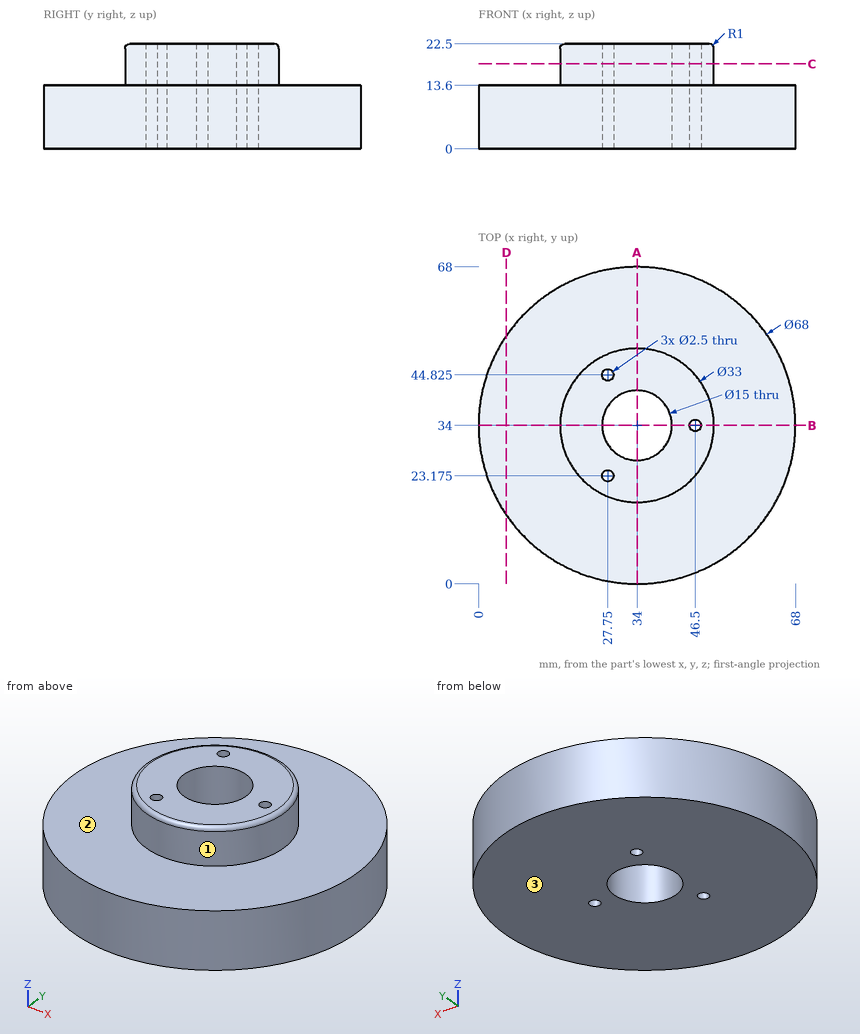
Can you work these out from the drawing? Everything is in mm from the part's minimum corner. Give positions to 0.01 mm unless a question says otherwise; leave off trailing zeros. Order: outer loops, then holes, each group sorted by start corner. A loop starts at its lowest first (then second) coordinate and runs counter-clockwise, first axis right, second up. Notation, with made-up numbers: (77.25, -7.75) -> (136.25, -7.75) arc R7 cw to (136.25, -3.75) -> close; hole circle Ø8 at (52, 0.25). An arc over 180 degrees is marked (long way). Return JSON: item names as keys, results as strings.
1. Imagine slicing it at A-A on x = 34. List the corners of the cut face in (y, z) for me.
Answer list:
{"outline": "(0, 0) -> (26.5, 0) -> (26.5, 22.5) -> (18.5, 22.5) arc R1 ccw to (17.5, 21.5) -> (17.5, 13.6) -> (0, 13.6) -> close; (41.5, 0) -> (68, 0) -> (68, 13.6) -> (50.5, 13.6) -> (50.5, 21.5) arc R1 ccw to (49.5, 22.5) -> (41.5, 22.5) -> close"}
2. Imagine slicing it at B-B on y = 34. List the corners of the cut face in (x, z) for me.
Answer list:
{"outline": "(0, 0) -> (26.5, 0) -> (26.5, 22.5) -> (18.5, 22.5) arc R1 ccw to (17.5, 21.5) -> (17.5, 13.6) -> (0, 13.6) -> close; (41.5, 0) -> (45.25, 0) -> (45.25, 22.5) -> (41.5, 22.5) -> close; (47.75, 0) -> (68, 0) -> (68, 13.6) -> (50.5, 13.6) -> (50.5, 21.5) arc R1 ccw to (49.5, 22.5) -> (47.75, 22.5) -> close"}
3. For pin 1 Ø1 at (y, z) = (37, 8.5) entering from +X; pin 2 Ø5 at (y, z) = (59.5, 14.5) entering from -X (1 decimal); pin 3 Ø3 at (x, z) = (7, 3.5) entering from +Y; pin 4 Ø4 at (x, y) = (27.75, 23.17) entering from -Z, each with a flat end and sliding along its axis, tell me the tip position at first contact or that it passes through.
Answer list:
{"pin 1": "stops at x = 67.91", "pin 2": "stops at x = 9.1", "pin 3": "stops at y = 56.49", "pin 4": "stops at z = 0"}
4. Imagine slicing it at D-D on x = 6. List the corners of the cut face in (y, z) for me, then the cut area to 3 significant figures.
Answer list:
{"outline": "(14.71, 0) -> (53.29, 0) -> (53.29, 13.6) -> (14.71, 13.6) -> close", "area": "525 mm2"}
5. Imagine slicing it at C-C on z = 18.25. Give the number of separate pieces and of enclosed holes in the cut face, then the cut area to 3 significant figures.
Answer list:
{"separate pieces": "1", "enclosed holes": "4", "area": "664 mm2"}
6. Thinking about a two-plate mould opening in Z: for the marked faces 1, 2 and 3, which applies, pulls with the +Z half, pulls with the -Z half, needs draft (parallel to the pull), parting line crosses it, or undercut?
Answer list:
{"face 1": "needs draft", "face 2": "pulls with the +Z half", "face 3": "pulls with the -Z half"}
7. I need wall thicknesses on line 1 (Y direction, x = 34, z = 12); line 2 (Y direction, x = 27.75, z = 4.75) (1 decimal); line 3 (Y direction, x = 27.75, z = 14.5) (1 decimal). Which ranges of each line are inside material? Lowest first, please. Write a range as from..to.
Answer list:
{"line 1": "y = 0..26.5, 41.5..68", "line 2": "y = 0.6..21.9, 24.4..29.9, 38.1..43.6, 46.1..67.4", "line 3": "y = 18.7..21.9, 24.4..29.9, 38.1..43.6, 46.1..49.3"}
